Autodesk Fusion 360 part; units mm, degrees
sketch "Boceto1" plane through (0, 0, 0) normal (0, 0, 1) x (1, 0, 0)
  line L0 (0, 0) -> (54, 0)
  line L1 (54, 0) -> (54, 28.5)
  line L2 (54, 28.5) -> (0, 28.5)
  line L3 (0, 28.5) -> (0, 0)
  dimension "d1" = 54
  dimension "d2" = 28.5
extrude "Extruir1" add sketch "Boceto1" along normal blind 11.5
fillet "Empalme1" radius 5 2 faces at (18, 9.5, 11.5) (18, 9.5, 0)
sketch "Boceto2" plane through (0, 0, 0) normal (-1, 0, 0) x (0, -1, 0)
  line L0 (-28.5, 5) -> (0, 5)
  line L1 (0, 5) -> (0, 6.5)
  line L2 (0, 6.5) -> (-28.5, 6.5)
  line L3 (-28.5, 6.5) -> (-28.5, 5)
  line L4 (-25, 2.75) -> (-5, 2.75)
  line L5 (-5, 2.75) -> (-5, 8.75)
  line L6 (-5, 8.75) -> (-25, 8.75)
  line L7 (-25, 8.75) -> (-25, 2.75)
  dimension "d7" = 5
  dimension "d8" = 20
  dimension "d9" = 6
  dimension "d10" = 2.75
extrude "Extruir2" add sketch "Boceto2" along normal blind 4 and the other way blind 1 contours L0 L2 L5 L7 | L0 L4 L5 L7 | L2 L5 L6 L7
chamfer "Chaflán1" distance 1 angle 45 5 edges at (-1.7326, 25, 8.75) (-1.7326, 25, 2.75) (-4, 15, 8.75) (-4, 15, 2.75) (-4, 25, 5.75)
equation "d10 = ( ( 11.5 - 6 ) / 2 ) * 1 mm"
Work out the finished part from the listing and answer in its coordinate system (mm). A direction names the side the tool comes from. Give positions to 0.01 mm unless a question says otherwise; leave off trailing zeros. Order: outer loops, then holes, each group sorted by start corner. A loop starts at its lowest first (then second) coordinate and runs counter-clockwise, first axis right, second up. Notation, with made-up numbers: (27.5, 17) -> (68.5, 17) arc R22 ccw to (68.5, 49) -> close; hole circle Ø7 at (-8, -32.5). An arc over 180 degrees is marked (long way). One line per item, written item: value.
Item 1: A tool of negligible diameter and unlimited length cuts with its end or side. For faces 1 (the flat face through (-1.26, 24.49, 3.24)), 2 (the flat face through (-1, 14, 8.75)), 3 (the flat face through (-1, 15, 2.75)), 4 (the flat face through (54, 14, 6)), from which of +Z, -Z, +X, -X, +Y, -Y can it reach the whole face along a straight path? Write none if from no direction.
Answer sheet:
face 1: -Z, -X, +Y
face 2: +Z, -X, +Y, -Y
face 3: -Z, -X, +Y, -Y
face 4: +Z, -Z, +X, +Y, -Y
Item 2: Flat-ended cylindrical pins translate along their axes: P1, Ø2, axis at x = 46, z = 10, coming from the -Y side; P2, Ø1.2, axis at y = 1.5, z = 6, coming from the -X side; P3, Ø1, axis at x = 34.5, z = 3, coming from the +Y side. Find the tip coordinate at first contact, or state that the pin passes through.
Answer sheet:
P1: y = 0.67
P2: x = 0
P3: y = 28.27
Item 3: Find section B-B, the plane x = 18.5. Give the vertices of the cut face in (y, z).
Answer sheet:
outline: (0, 5) arc R5 ccw to (5, 0) -> (23.5, 0) arc R5 ccw to (28.5, 5) -> (28.5, 6.5) arc R5 ccw to (23.5, 11.5) -> (5, 11.5) arc R5 ccw to (0, 6.5) -> close
Item 4: Find section C-C, the plane z = 2. Give the vertices of the cut face in (x, y).
Answer sheet:
outline: (1, 1) -> (53, 1) -> (53, 27.5) -> (1, 27.5) -> close
Item 5: Find section D-D, the plane y = 26.5. Give the vertices of the cut face in (x, z), plus the area to 3 significant figures.
Answer sheet:
outline: (0, 5) arc R5 ccw to (2, 1) -> (52, 1) arc R5 ccw to (54, 5) -> (54, 6.5) arc R5 ccw to (52, 10.5) -> (2, 10.5) arc R5 ccw to (0, 6.5) -> close
area: 503 mm²
Item 6: Find section A-A, the plane y = 6. Give the vertices of the cut face in (x, z).
Answer sheet:
outline: (-4, 3.75) -> (-3, 2.75) -> (0.53, 2.75) arc R5 ccw to (5, 0) -> (49, 0) arc R5 ccw to (54, 5) -> (54, 6.5) arc R5 ccw to (49, 11.5) -> (5, 11.5) arc R5 ccw to (0.53, 8.75) -> (-3, 8.75) -> (-4, 7.75) -> close
Item 7: Straight lines are drawn through the part: probe 1 along Y at (x, z) = (-1, 6); probe 2 along X at (y, z) = (4.75, 5.25); probe 3 along X at (y, z) = (13.75, 4.5). For each, find the intervals that lie inside material, in ascending order.
Answer sheet:
probe 1: 5 to 25
probe 2: 0 to 54
probe 3: -4 to 53.97
